from build123d import *

# Parameters (mm, degrees)
SCHIZZO1_R                   = 0.75
ESTRUSIONE_ESTRUSIONE1_DEPTH = 3
TAGLIO_ESTRUSIONE2_START     = 0.5
TAGLIO_ESTRUSIONE2_OUTLINE_R = 0.75
TAGLIO_ESTRUSIONE2_DEPTH     = 2
RACCORDO1_R                  = 0.5


with BuildPart() as part:
    # Schizzo1 → Estrusione-Estrusione1 (new body)
    with BuildSketch(Plane.XY):
        with BuildLine():
            Line((1.335883711, 7), (-5.5, 7))
            ThreePointArc((-5.5, 7), (-6.207106781, 6.707106781), (-6.5, 6))
            Line((-6.5, 6), (-6.5, 1))
            ThreePointArc((-6.5, 1), (-6.792893219, 0.292893219), (-7.5, 0))
            Line((-7.5, 0), (-16.5, 0))
            Line((-16.5, 0), (-16.5, -3))
            ThreePointArc((-16.5, -3), (0.101782453, -2.23760178), (16.521096634, 0.332719886))
            ThreePointArc((16.521096634, 0.332719886), (18.472600065, 3.146927603), (15.784267214, 5.268482974))
            ThreePointArc((15.784267214, 5.268482974), (8.632526621, 5.382625954), (1.653331613, 6.948275714))
            ThreePointArc((1.653331613, 6.948275714), (1.496700822, 6.986984223), (1.335883711, 7))
        make_face()
        with Locations((0, 4)):
            Circle(SCHIZZO1_R, mode=Mode.SUBTRACT)
        with Locations((16, 2.777808494)):
            Circle(SCHIZZO1_R, mode=Mode.SUBTRACT)
    extrude(amount=ESTRUSIONE_ESTRUSIONE1_DEPTH)

    # Taglio-Estrusione2: read off the stored shape, not the designer's step
    # Taglio-Estrusione2 outline → Taglio-Estrusione2 (cut)
    with BuildSketch(Plane.XY.offset(TAGLIO_ESTRUSIONE2_START)):
        with BuildLine():
            ThreePointArc((-16.5, -2.5), (0.79291183, -1.666252109), (17.878837946, 1.128575953))
            ThreePointArc((17.878837946, 1.128575953), (18.230736925, 3.906441637), (15.784267214, 5.268482974))
            ThreePointArc((15.784267214, 5.268482974), (8.632526621, 5.382625954), (1.653331613, 6.948275714))
            ThreePointArc((1.653331613, 6.948275714), (1.496700822, 6.986984223), (1.335883711, 7))
            Line((1.335883711, 7), (-5.5, 7))
            ThreePointArc((-5.5, 7), (-6.207106781, 6.707106781), (-6.5, 6))
            Line((-6.5, 6), (-6.5, 1))
            ThreePointArc((-6.5, 1), (-6.792893219, 0.292893219), (-7.5, 0))
            Line((-7.5, 0), (-16.5, 0))
            Line((-16.5, 0), (-16.5, -2.5))
        make_face()
        with Locations((0, 4)):
            Circle(TAGLIO_ESTRUSIONE2_OUTLINE_R, mode=Mode.SUBTRACT)
        with Locations((16, 2.777808494)):
            Circle(TAGLIO_ESTRUSIONE2_OUTLINE_R, mode=Mode.SUBTRACT)
    extrude(amount=TAGLIO_ESTRUSIONE2_DEPTH, mode=Mode.SUBTRACT)

    # Raccordo1
    # the kernel refuses this fillet: 0.5 mm, written as the material it takes off along each edge
    with BuildSketch(Plane(origin=(-15.161578714, 148.994107216, 0), x_dir=(-0.017028442214045383, -0.9998550055661886, 0), z_dir=(-0.9998550055661886, 0.017028442214045383, 0))) as raccordo1_piece_1:
        with BuildLine():
            CenterArc((152 - RACCORDO1_R, RACCORDO1_R), RACCORDO1_R, 270, 90)
            Line((152, RACCORDO1_R), (152, 0))
            Line((152, 0), (152 - RACCORDO1_R, 0))
        make_face()
    revolve(axis=Axis((-15.161578714, 148.994107216, 0), (0, 0, 1)), revolution_arc=13.807590381, mode=Mode.SUBTRACT)
    with BuildSketch(Plane(origin=(-15.161578714, 148.994107216, 3), x_dir=(-0.017028442214045383, -0.9998550055661886, 0), z_dir=(-0.9998550055661886, 0.017028442214045383, 0))) as raccordo1_piece_2:
        with BuildLine():
            CenterArc((152 - RACCORDO1_R, -RACCORDO1_R), RACCORDO1_R, 0, 90)
            Line((152 - RACCORDO1_R, 0), (152, 0))
            Line((152, 0), (152, -RACCORDO1_R))
        make_face()
    revolve(axis=Axis((-15.161578714, 148.994107216, 3), (0, 0, 1)), revolution_arc=13.807590381, mode=Mode.SUBTRACT)


solid = part.part
Verification items for the finished model (mm, model axes). A direction names the side the tool comes from. Give positions to 0.01 mm unless a question says otherwise; leave off trailing zeros. Write each loop counter-clockwise with the first axis right and the second up, starting at its lowest first coordinate (ties: lowest second). Pieces come first, ordered by that corner, then holes. Notation, with made-up numbers: M 44.25,41 L 60.25,41 A17 ccw 60.25,46 Z; hole C 40.5,22.25 d3. An arc over 180 degrees is marked long. Use CSV: the item, a comma, the result in double quotes.
1) Access from +Z, -Z, +X, -X, +Y, -Y to the whole of each face (thin tool, end or side, straight path). Record for faces 1 (the face through (1, 2, 0.5)), 2 (the face through (-0.163, 3.268, 0.246)).
Final values:
face 1,"-X, +Y"
face 2,"+Z, -Z"
2) Cross-section at A-A (y = 4). Enter the section's corners in (x, z), plus the area to 3 significant figures.
Final values:
outline,"M -6.5,0 L -0.75,0 L -0.75,0.5 L -6.5,0.5 Z; M -6.5,2.5 L -0.75,2.5 L -0.75,3 L -6.5,3 Z; M 0.75,0 L 18.18,0 L 18.18,0.5 L 0.75,0.5 Z; M 0.75,2.5 L 18.18,2.5 L 18.18,3 L 0.75,3 Z"
area,"23.2 mm²"
3) Go/stop test with flat-tipped pins: pin 1 Ø4 at (x, y) = (-10, 3) entering from -Z; pin 2 Ø1.5 at (x, z) = (14.5, 2) entering from +Y; pin 3 Ø0.6 at (y, z) = (2.5, 0.5) entering from -X. Record where each tip stops, or that it passes through.
Final values:
pin 1,"through"
pin 2,"y = 5.21"
pin 3,"x = -6.5"
4) Release check for a two-part mould opening along X. For faces 3 (the face through (1, 2, 3)), 4 (the face through (15.25, 2.81, 2.75)), 5 (the face through (-6.785, 0.301, 0.246)) record: released by +X, released by -X, zero draft, split by the parting line, or undercut.
Final values:
face 3,"zero draft"
face 4,"undercut"
face 5,"released by -X"
5) Cross-section at B-B (z = 2.2). Enter the section's corners in (x, y).
Final values:
outline,"M -16.5,-3 A152 ccw 16.52,0.33 A2.5 ccw 17.88,1.13 A152 cw -16.5,-2.5 Z"
